Model file for the job. Use its own axes, mm. Coordinates: 2 decimals unless noted, no trailing zeros. Write each loop counter-clockwise with the first axis right and the second up, starting at its lowest first coordinate (ties: lowest second). Pieces come first, ordered by that corner, then holes. Notation, with made-up numbers: M 50,47.5 L 99,47.5 A25 cw 99,65.5 Z; hole C -4.75,87.5 d5. An arc over 180 degrees is marked long. One line per question, with ' | ' between items. Start each with the question number.
(1) Cut at C-C (x = 48.5). Write the cut outline in (y, z), plus the area to 3 significant figures.
(2) Wall check: probe 1 along X at (y, z) = (-19.5, 3.5); probe 2 along Y at (x, z) = (14, 13.75); probe 3 along X at (y, z) = (93, 17). Give the ranges that are in metal, low to high.
(3) Cut at A-A (z = 7.25). Count the separate pieces of the cut face and the enclosed holes in it, plus the area to 3 significant figures.
(4) Flat gauge pins, fed straight in: pin 1 Ø3 at (x, y) = (21.66, 179.3) entering from +Z (3 decimals); pin 2 Ø1 at (y, z) = (103.5, 16.5) entering from +X; pin 3 Ø12 at (y, z) = (74, 16.5) entering from -X; pin 4 Ø5 at (x, z) = (-10, 6) entering from +Y. Where does each tip first touch, or does it go through?
(5) Cut at B-B (y = 82.5). Write the cut outline in (x, z), plus the area to 3 significant figures.
from build123d import *

# Parameters (mm, degrees)
BOSS_EXTRUDE1_DEPTH = 20
SKETCH2_R           = 3.5
SKETCH2_R_2         = 2
CUT_EXTRUDE6_DEPTH  = 208.432644896
SKETCH4_R           = 3.5
SKETCH4_R_2         = 2
CUT_EXTRUDE8_DEPTH  = 208.432644896


with BuildPart() as part:
    # Sketch1 → Boss-Extrude1 (new body)
    with BuildSketch(Plane.XY):
        with BuildLine():
            ThreePointArc((-42.5, -44.96942423), (0.373210889, -87.467785535), (42.493445347, -44.223031232))
            ThreePointArc((42.493445347, -44.223031232), (58.699206053, 32.335771546), (42.750578742, 108.948552787))
            ThreePointArc((42.750578742, 108.948552787), (33.960784088, 136.689765999), (30.650815647, 165.601346886))
            ThreePointArc((30.650815647, 165.601346886), (-2.129568534, 197.52932265), (-34.344171972, 165.03057577))
            ThreePointArc((-34.344171972, 165.03057577), (-37.145879301, 136.065323543), (-45.447121923, 108.174020751))
            ThreePointArc((-45.447121923, 108.174020751), (-60.04780144, 31.292962484), (-42.5, -44.96942423))
        make_face()
    extrude(amount=BOSS_EXTRUDE1_DEPTH)

    # Sketch2 → Cut-Extrude6 (cut, through all)
    with BuildSketch(Plane.XY.offset(20)):
        with Locations((-1.844171972, 155.798868961)):
            Circle(SKETCH2_R)
        with Locations((21.655828028, 179.298868961)):
            Circle(SKETCH2_R_2)
        with Locations((-25.344171972, 179.298868961)):
            Circle(SKETCH2_R_2)
        with Locations((21.655828028, 132.298868961)):
            Circle(SKETCH2_R_2)
        with Locations((-25.344171972, 132.298868961)):
            Circle(SKETCH2_R_2)
    extrude(amount=-CUT_EXTRUDE6_DEPTH, mode=Mode.SUBTRACT)

    # Sketch4 → Cut-Extrude8 (cut, through all)
    with BuildSketch(Plane.XY.offset(20)):
        with Locations((1.132601083, -41.747329739)):
            Circle(SKETCH4_R)
        with Locations((24.632601083, -18.247329739)):
            Circle(SKETCH4_R_2)
        with Locations((-22.367398917, -18.247329739)):
            Circle(SKETCH4_R_2)
        with Locations((24.632601083, -65.247329739)):
            Circle(SKETCH4_R_2)
        with Locations((-22.367398917, -65.247329739)):
            Circle(SKETCH4_R_2)
    extrude(amount=-CUT_EXTRUDE8_DEPTH, mode=Mode.SUBTRACT)


solid = part.part
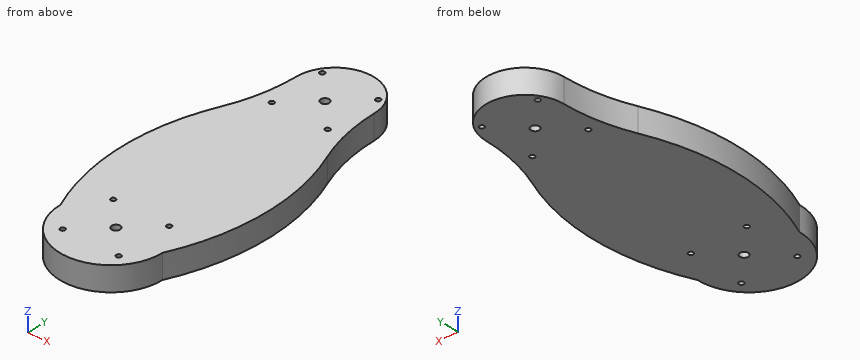
Filled in:
1) outline: M -28.83,0 L 94.15,0 L 94.15,20 L -28.83,20 Z | area: 2,460 mm²
2) probe 1: -52.13 to -23.93, -20.81 to 23.07, 26.19 to 51.42 | probe 2: -85.1 to 193.41 | probe 3: -51.02 to 48.89
3) separate pieces: 1 | enclosed holes: 10 | area: 25,000 mm²
4) pin 1: through | pin 2: x = 45.23 | pin 3: x = -57.19 | pin 4: y = 197.03
5) outline: M -54.05,0 L 52.06,0 L 52.06,20 L -54.05,20 Z | area: 2,120 mm²
